Geometry: final body of the model. Coordinates: model frame, mm. A direction names the side the tool comes from. Coordinates: 2 decimals unless noted, no trailing zeros. Loops run counter-clockwise (first coordinate to the right, second up) from the corner with the lowest first, then second, coordinate; pieces in that order, holes last. Notation, with made-up numbers: M 66,85 L 121,85 A6 cw 121,91 Z; hole C 61,76.25 d7. An arc over 180 degrees is marked long. Write item = value, one per line. Start each with the question number.
```python
from build123d import *

# Parameters (mm, degrees)
F2_R     = 2.54
F3_DEPTH = 9.6022
F4_SIZE  = 1.5
F5_SIZE2 = 2.5
F5_SIZE  = 2


with BuildPart() as f1:
    # F0 (on Front) → F1 (revolve)
    with BuildSketch(Plane.XZ):
        Polygon((31.75, -5.978718), (31.75, -2.727518), (18.161, -2.727518), (18.161, 3.622482), (15, 3.622482), (15, -8.179607), (10.922, -8.179607), (10.922, -12.328718), (18.161, -12.328718), (18.161, -5.978718), align=None)
    revolve(axis=Axis((0, 0, -5.153181), (0, 0, -1)))

    # F2 (on face) → F3 (cut, through all)
    with BuildSketch(Plane.XY.offset(-2.727518)):
        with Locations((26.3906, 0)):
            Circle(F2_R)
        with Locations((-26.3906, 0)):
            Circle(F2_R)
    extrude(amount=-F3_DEPTH, mode=Mode.SUBTRACT)

    # F4
    f4_edges = [f1.edges().sort_by_distance(p)[0] for p in [
        (-18.161, 0, -12.328718),
    ]]
    chamfer(f4_edges, length=F4_SIZE)

    # F5
    f5_edges = [f1.edges().sort_by_distance(p)[0] for p in [
        (-15, 0, 3.622482),
    ]]
    chamfer(f5_edges, length=F5_SIZE, length2=F5_SIZE2)


solid = f1.part
```
Item 1: Section query C-C (z = -9.25). Return the cut outline in (x, y), plus the area to 3 significant figures.
Item 2: Section query A-A (y = 0). Count the separate pieces of the cut face and the enclosed holes in it, plus the area to 3 significant figures.
Item 3: First-contact query: pin 1 (2 mm diameter, centred on x = 21, y = -7.5, fed in from -Z); pin 2 (4.5 mm diameter, centred on x = -26.39, y = 0, fed in from +Z); pin 3 (1.5 mm diameter, centred on x = -14.5, z = 0.5, fed in from +Y); pin 4 (2 mm diameter, centred on x = -21.5, z = -5, fed in from -Y). Flat tips, straight axial feed; report the tip coordinate or a pass-through.
Item 4: Section query B-B (x = 0). Return the cut outline in (y, z), plus the area to 3 significant figures.
Item 5: Pull-direction query (X, two-part tool) for faces 1 (the flat face through (1.04, 11.04, -8.18)), 2 (the flat face through (-14.9, -9.5, 3.622)), 3 (the cylindrical face through (-6.883, 30.995, -4.33)); classes: released by +X, released by -X, zero draft, split by the parting line, or undercut.
Item 6: Section query D-D (z = -4). Return the cut outline in (x, y), plus the area to 3 significant figures.
Item 7: Reachability of faces 4 (the cylindrical face through (10.418, -3.281, -10.283)), 5 (the cylindrical face through (9.763, -15.313, 0.492)), 6 (the cylindrical face through (9.763, -15.313, -8.37)) from +Z, -Z, +X, -X, +Y, -Y: full face, straight path, thin tool, end or side. Return the list, or none.
Item 8: Line query: line 1 (Y direction, x = 0, z = -1); line 2 (Y direction, x = 0, z = -9.75); line 3 (Z direction, x = 25.5, y = -3.5). Output: solid intervals per line, ascending. Write a range as from..to.
Verdict:
q1.outline = C 0,0 d36.32; hole C 0,0 d21.84
q1.area = 661 mm2
q2.separate_pieces = 4
q2.enclosed_holes = 0
q2.area = 183 mm2
q3.pin_1 = -5.98
q3.pin_2 = through
q3.pin_3 = 11.86
q3.pin_4 = -24.24
q4.outline = M -31.75,-5.98 L -18.16,-5.98 L -18.16,-10.83 L -16.66,-12.33 L -10.92,-12.33 L -10.92,-8.18 L -15,-8.18 L -15,1.62 L -17.5,3.62 L -18.16,3.62 L -18.16,-2.73 L -31.75,-2.73 Z; M 10.92,-12.33 L 16.66,-12.33 L 18.16,-10.83 L 18.16,-5.98 L 31.75,-5.98 L 31.75,-2.73 L 18.16,-2.73 L 18.16,3.62 L 17.5,3.62 L 15,1.62 L 15,-8.18 L 10.92,-8.18 Z
q4.area = 216 mm2
q5.face_1 = undercut
q5.face_2 = zero draft
q5.face_3 = split by the parting line
q6.outline = C 0,0 d63.5; hole C -26.39,0 d5.08; hole C 0,0 d30; hole C 26.39,0 d5.08
q6.area = 2,420 mm2
q7.face_4 = +Z, -Z
q7.face_5 = +Z
q7.face_6 = -Z
q8.line_1 = -18.16..-15, 15..18.16
q8.line_2 = -18.16..-10.92, 10.92..18.16
q8.line_3 = -5.98..-2.73
